```python
from build123d import *

# Parameters (mm, degrees)
SKETCH_1_R               = 13.5
SKETCH_1_R_2             = 10.5
EXTRUDE_1_DEPTH          = 20
EXTRUDE_2_REACH          = 43.286
EXTRUDE_2_END_RADIUS     = 13.5
SKETCH_5_W               = 27
SKETCH_5_H               = 20
CUT_EXTRUDE_2_DEPTH      = 32.340867888
CUT_EXTRUDE_2_DEPTH_BACK = 32.340867888
SKETCH_2_R               = 3.2
SKETCH_6_W               = 4
SKETCH_6_H               = 20
EXTRUDE_4_DEPTH          = 5
FILLET_1_R               = 5
SKETCH_7_R               = 1.9
CUT_EXTRUDE_3_DEPTH      = 5


with BuildPart() as part:
    # 草图1 → 凸台-拉伸1 (new body)
    with BuildSketch(Plane(origin=(0, 0, 0), x_dir=(1, 0, 0), z_dir=(0, 1, 0))):
        with Locations(Location((0, 0, 0), (0, 0, 270))):
            Circle(SKETCH_1_R)
        with Locations(Location((0, 0, 0), (0, 0, 270))):
            Circle(SKETCH_1_R_2, mode=Mode.SUBTRACT)
    extrude(amount=EXTRUDE_1_DEPTH)

    # 凸台-拉伸2: up to this cylinder (the profile starts outside it)
    extrude_2_end = Plane(origin=(0, 10, 0), z_dir=(0, -1, 0)) * Cylinder(EXTRUDE_2_END_RADIUS, 114.572, mode=Mode.PRIVATE)
    # 草图5 → 凸台-拉伸2 (add, up to the surface)
    with BuildSketch(Plane.XY.offset(20), mode=Mode.PRIVATE) as extrude_2_sk1:
        with Locations((0, 10)):
            Rectangle(SKETCH_5_W, SKETCH_5_H)
    extrude_2_tool1 = extrude(extrude_2_sk1.sketch, amount=-EXTRUDE_2_REACH, mode=Mode.PRIVATE) - extrude_2_end
    add(extrude_2_tool1.solids().sort_by_distance((0, 10, 20))[0])

    # 草图2 → 切除-拉伸2 (cut, two sides: drawn at the far end of the back side and taken through both)
    with BuildSketch(Plane(origin=(0, 0, 0), x_dir=(0, 0, -1), z_dir=(1, 0, 0)).offset(-CUT_EXTRUDE_2_DEPTH_BACK)):
        with Locations((0, 10)):
            Circle(SKETCH_2_R)
    extrude(amount=CUT_EXTRUDE_2_DEPTH + CUT_EXTRUDE_2_DEPTH_BACK, mode=Mode.SUBTRACT)

    # 草图6 → 凸台-拉伸4 (add)
    with BuildSketch(Plane.XY.offset(20)):
        with Locations((15.5, 10)):
            Rectangle(SKETCH_6_W, SKETCH_6_H)
        with Locations((11.5, 10)):
            Rectangle(SKETCH_6_W, SKETCH_6_H)
        with Locations((-11.5, 10)):
            Rectangle(SKETCH_6_W, SKETCH_6_H)
        with Locations((-15.5, 10)):
            Rectangle(SKETCH_6_W, SKETCH_6_H)
    extrude(amount=EXTRUDE_4_DEPTH)

    # 圆角1
    # the kernel refuses this fillet: 5 mm, written as the material it adds along each edge
    with BuildSketch(Plane(origin=(13.5, 20, 20), x_dir=(0, 0, -1), z_dir=(0, -1, 0)), Plane(origin=(-13.5, 0, 20), x_dir=(0, 0, -1), z_dir=(0, 1, 0))) as fillet_1_piece_1:
        with BuildLine():
            CenterArc((4.898979486, 5), FILLET_1_R, 191.536959033, 78.463040967)
            Line((0, 4), (-0.09797959, 3.98))
            ThreePointArc((-0.09797959, 3.98), (-0.1, 2), (-0.1, 0))
            Line((-0.1, 0), (0, -0.1))
            Line((0, -0.1), (4.898979486, -0.1))
            Line((4.898979486, -0.1), (4.898979486, 0))
        make_face()
    extrude(amount=20)

    # 草图7 → 切除-拉伸3 (cut)
    with BuildSketch(Plane.XY.offset(25)):
        with Locations((13.5, 10)):
            Circle(SKETCH_7_R)
        with Locations(Location((-13.5, 10, 0), (0, 0, 180))):
            Circle(SKETCH_7_R)
    extrude(amount=-CUT_EXTRUDE_3_DEPTH, mode=Mode.SUBTRACT)


solid = part.part
```
Could you check a few things on this model? Use its own coordinates, in mm. A direction names the side the tool comes from. Coordinates: 2 decimals unless noted, no trailing zeros. Loops run counter-clockwise (first coordinate to the right, second up) from the corner with the lowest first, then second, coordinate; pieces in that order, holes last.
1) Imagine slicing it at A-A (z = 21.5). List the corners of the cut face in (x, y) for me, and give its area (3 significant figures).
Reported:
outline: (-17.5, 0) - (-9.5, 0) - (-9.5, 20) - (-17.5, 20) - close; (9.5, 0) - (17.5, 0) - (17.5, 20) - (9.5, 20) - close; hole circle Ø3.8 at (-13.5, 10); hole circle Ø3.8 at (13.5, 10)
area: 297 mm2
2) Please list where these lines run through material, in increasing order: line 1 along Y through (x, z) = (-13.5, 21.4); line 2 along Y through (x, z) = (12, 0); line 3 along X through (y, z) = (9.5, 23).
Reported:
line 1: y = 0 to 8.1, 11.9 to 20
line 2: y = 0 to 6.8, 13.2 to 20
line 3: x = -17.5 to -15.33, -11.67 to -9.5, 9.5 to 11.67, 15.33 to 17.5
3) Imagine slicing it at D-D (y = 14.25). List the corners of the cut face in (x, z) for me, and give its area (3 significant figures).
Reported:
outline: (-17.5, 20) arc R5 cw to (-13.5, 15.1) - (-13.5, 0) arc R13.5 ccw to (13.5, 0) - (13.5, 15.1) arc R5 cw to (17.5, 20) - (17.5, 25) - (9.5, 25) - (9.5, 20) - (-9.5, 20) - (-9.5, 25) - (-17.5, 25) - close; hole circle Ø21 at (0, 0)
area: 570 mm2
4) Imagine slicing it at B-B (x = 0). List the corners of the cut face in (y, z) for me.
Reported:
outline: (0, -13.5) - (20, -13.5) - (20, -10.5) - (0, -10.5) - close; (0, 10.5) - (20, 10.5) - (20, 20) - (0, 20) - close
5) Thinking about a two-plate mould opening in Z: for faces 5 (the face through (4, 20, 10)), 6 (the face through (-11.772, 8.053, 2.539)), 7 (the face through (13, 12, 25)), which applies, released by +Z, released by -Z, zero draft, split by the parting line, or undercut?
Reported:
face 5: zero draft
face 6: undercut
face 7: released by +Z
6) Imagine slicing it at C-C (z = -10). List the corners of the cut face in (x, y) for me, and give its area (3 significant figures).
Reported:
outline: (-9.07, 0) - (-3.2, 0) - (-3.2, 20) - (-9.07, 20) - close; (3.2, 0) - (9.07, 0) - (9.07, 20) - (3.2, 20) - close
area: 235 mm2
7) Will these pins go through, and if not, where does the flat tip stop? pin 1 Ø8 at (x, y) = (0, 4.5) entering from +Z; pin 2 Ø7.5 at (y, z) = (11.5, 11.5) entering from +X; pin 3 Ø4 at (y, z) = (7, 13.5) entering from -X.
Reported:
pin 1: stops at z = 20
pin 2: stops at x = 13.5
pin 3: stops at x = -13.52
8) Which directions (+Z, -Z, +X, -X, +Y, -Y) give clear straight access to the entire face, cutting with the end or side of a thin tool? Please do faces 1 (the face through (11.6, 10.08, 22.54)), 2 (the face through (13.5, 10, 8)), 3 (the face through (-13.5, 10, 8)), 4 (the face through (9.5, 10, 22)).
Reported:
face 1: +Z
face 2: -Z, +X, +Y, -Y
face 3: -Z, -X, +Y, -Y
face 4: +Z, +Y, -Y
